```python
from build123d import *

# Parameters (mm, degrees)
BOSS_EXTRUDE1_DEPTH = 9.525
BOSS_EXTRUDE2_DEPTH = 3.175
BOSS_EXTRUDE3_START = -12.7
BOSS_EXTRUDE3_DEPTH = 3.175


with BuildPart() as part:
    # Sketch1 → Boss-Extrude1 (new body)
    with BuildSketch(Plane.XY):
        with BuildLine():
            Line((-6.9088, 0), (6.9088, 0))
            ThreePointArc((6.9088, 0), (11.229329629, 0.569673931), (15.254541002, 2.239757184))
            Line((15.254541002, 2.239757184), (12.609003955, 2.706236743))
            ThreePointArc((12.609003955, 2.706236743), (9.813274868, 1.869826819), (6.9088, 1.5875))
            Line((6.9088, 1.5875), (-6.9088, 1.5875))
            ThreePointArc((-6.9088, 1.5875), (-8.731329847, 1.950023726), (-10.276396045, 2.982403955))
            Line((-10.276396045, 2.982403955), (-11.398928061, 1.859871939))
            ThreePointArc((-11.398928061, 1.859871939), (-9.338839796, 0.483364969), (-6.9088, 0))
        make_face()
    extrude(amount=BOSS_EXTRUDE1_DEPTH)

    # Sketch2 → Boss-Extrude2 (add)
    with BuildSketch(Plane.XY.offset(9.525)):
        with BuildLine():
            Line((6.9088, 0), (6.9088, 1.5875))
            Line((6.9088, 1.5875), (-6.9088, 1.5875))
            ThreePointArc((-6.9088, 1.5875), (-8.731329847, 1.950023726), (-10.276396045, 2.982403955))
            Line((-10.276396045, 2.982403955), (-11.398928061, 1.859871939))
            ThreePointArc((-11.398928061, 1.859871939), (-9.338839796, 0.483364969), (-6.9088, 0))
            Line((-6.9088, 0), (6.9088, 0))
        make_face()
    extrude(amount=BOSS_EXTRUDE2_DEPTH)

    # Sketch2<2> → Boss-Extrude3 (add)
    with BuildSketch(Plane.XY.offset(9.525).offset(BOSS_EXTRUDE3_START)):
        with BuildLine():
            Line((-6.9088, 0), (6.9088, 0))
            Line((6.9088, 0), (6.9088, 1.5875))
            Line((6.9088, 1.5875), (-6.9088, 1.5875))
            ThreePointArc((-6.9088, 1.5875), (-8.731329847, 1.950023726), (-10.276396045, 2.982403955))
            Line((-10.276396045, 2.982403955), (-11.398928061, 1.859871939))
            ThreePointArc((-11.398928061, 1.859871939), (-9.338839796, 0.483364969), (-6.9088, 0))
        make_face()
    extrude(amount=BOSS_EXTRUDE3_DEPTH)


solid = part.part
```
Geometry check sheet. Reference: the model listing, model coordinates, mm. A direction names the side the tool comes from. Coordinates: 2 decimals unless noted, no trailing zeros. Order: outer loops, then holes, each group sorted by start corner. A loop starts at its lowest first (then second) coordinate and runs counter-clockwise, first axis right, second up.
Item 1: Depth check by flat-ended pin: pin 1 (1.3 mm diameter, centred on y = 1, z = 10.5, fed in from +X); pin 2 (8 mm diameter, centred on x = -4.5, z = -0.5, fed in from +Y); pin 3 (1 mm diameter, centred on y = 2.5, z = 1.5, fed in from -X). Enter the tip coordinate at first touch or a pass-through.
Item 2: Section check B-B (x = 4.5). Enter the section's corners in (y, z) (1 decimal), plus the area to 3 significant figures.
Item 3: Scan lines: line 1 along Y through (x, z) = (3.75, 6); line 2 along Z through (x, y) = (7.75, 0.25) (3 decimals); line 3 along X through (y, z) = (0.65, -0.5). Record each from-to range of solid material in increasing order.
Item 4: Tool access check on faces 1 (the flat face through (11, 1, 9.525)), 2 (the cylindrical face through (-8.71, 1.94, 4.65)), 3 (the flat face through (-2, 1, -3.175)), 4 (the flat face through (6.909, 1, -2)). Record the directions out of +Z, -Z, +X, -X, +Y, -Y that give a thin tool (end or side, any length) a straight path to the whole face; none if there is none.
Item 5: Section check C-C (y = 0.75). Enter the section's corners in (x, z) (3 decimals).
Check sheet entries:
1. pin 1: stops at x = 6.91
1. pin 2: stops at y = 1.86
1. pin 3: stops at x = -11.26
2. outline: (0, -3.2) - (1.6, -3.2) - (1.6, 12.7) - (0, 12.7) - close
2. area: 25.2 mm2
3. line 1: y = 0 to 1.59
3. line 2: z = 0 to 9.525
3. line 3: x = -9.71 to 6.91
4. face 1: +Z, +X, +Y, -Y
4. face 2: +Z, -Z, +Y
4. face 3: -Z, +X, -X, +Y, -Y
4. face 4: -Z, +X, +Y, -Y
5. outline: (-9.903, -3.175) - (6.909, -3.175) - (6.909, 0) - (11.853, 0) - (11.853, 9.525) - (6.909, 9.525) - (6.909, 12.7) - (-9.903, 12.7) - close
